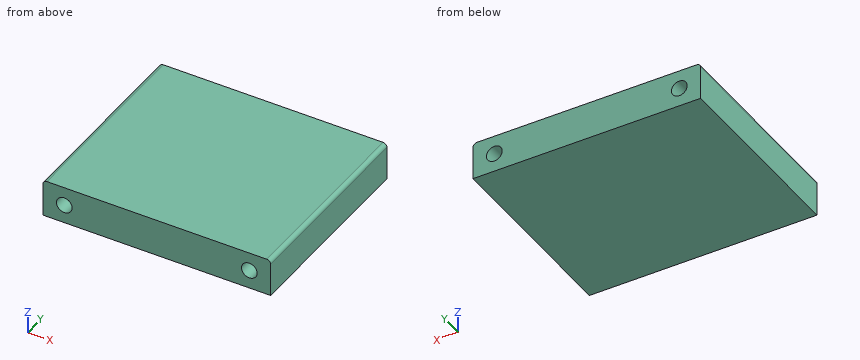
```python
from build123d import *

# Parameters (mm, degrees)
SKETCH_W  = 58
SKETCH_H  = 9.52
SKETCH_R  = 2
PAD_DEPTH = 50
FILLET_R  = 1


with BuildPart() as part:
    # Sketch → Pad (new body)
    with BuildSketch(Plane.XZ):
        Rectangle(SKETCH_W, SKETCH_H)
        with Locations((-23.57, 0)):
            Circle(SKETCH_R, mode=Mode.SUBTRACT)
        with Locations((23.57, 0)):
            Circle(SKETCH_R, mode=Mode.SUBTRACT)
    extrude(amount=PAD_DEPTH)

    # Fillet
    fillet_edges = [part.edges().sort_by_distance(p)[0] for p in [
        (29, -25, 4.76),
        (-29, -25, 4.76),
    ]]
    fillet(fillet_edges, radius=FILLET_R)


solid = part.part
```
Geometry check sheet. Reference: the model listing, model coordinates, mm. Round coordinates to 2 decimals unless told otherwise and drop trailing zeros. Order: outer loops, then holes, each group sorted by start corner. A loop starts at its lowest first (then second) coordinate and runs counter-clockwise, first axis right, second up. Notation, with made-up numbers: (-33.5, 52.25) -> (24.5, 52.25) arc R22 cw to (24.5, 73.25) -> close; hole circle Ø1 at (-24.5, -27.75). An arc over 180 degrees is marked (long way). Return JSON: item names as keys, results as strings. Group by question number.
Q1. Gauge pin test, flat end, axial feed: pin 1 (5 mm diameter, centred on x = -23, z = -1, fed in from -Y). Record the tip position at first contact, or that the pin passes through.
Q2. Section check B-B, the plane y = -10. Record the boundary of the cut face in (x, z), plus the area to 3 significant figures.
Q3. Section check A-A, the plane x = -23.57. Record the boundary of the cut face in (y, z), plus the area to 3 significant figures.
Q4. Material ranges on probe 1 along Z at (x, y) = (23.57, -27); probe 2 along X at (y, z) = (-20, -1); probe 3 along Z at (x, y) = (23, -9), recorded low to high. Write a range as from..to.
Numbers:
{
 "1": {"pin 1": "y = -50"},
 "2": {"outline": "(-29, -4.76) -> (29, -4.76) -> (29, 3.76) arc R1 ccw to (28, 4.76) -> (-28, 4.76) arc R1 ccw to (-29, 3.76) -> close; hole circle Ø4 at (-23.57, 0); hole circle Ø4 at (23.57, 0)", "area": "527 mm^2"},
 "3": {"outline": "(-50, -4.76) -> (0, -4.76) -> (0, -2) -> (-50, -2) -> close; (-50, 2) -> (0, 2) -> (0, 4.76) -> (-50, 4.76) -> close", "area": "276 mm^2"},
 "4": {"probe 1": "-4.76..-2, 2..4.76", "probe 2": "-29..-25.3, -21.84..21.84, 25.3..29", "probe 3": "-4.76..-1.92, 1.92..4.76"}
}
